Check sheet for the modelled part. Datum: model origin and axes. Units: mm. Face numbers are marked on the shaded views. A direction names the side the tool comes from. Round coordinates to 2 decimals unless told otherwise and drop trailing zeros. One line per item, written item: value.
from build123d import *

# Parameters (mm, degrees)
CUT_EXTRUDE1_DEPTH      = 5
CUT_EXTRUDE1_DEPTH_BACK = 20.845866419
SKETCH2_W               = 7
SKETCH2_H               = 11
SKETCH2_H_2             = 13
CUT_EXTRUDE2_DEPTH      = 20.845866419
CUT_EXTRUDE2_DEPTH_BACK = 20.845866419
SKETCH3_R               = 1
CUT_EXTRUDE4_START      = -7.009047527
CUT_EXTRUDE4_DEPTH      = 14.018095848
SKETCH6_R               = 0.5
CUT_EXTRUDE5_DEPTH      = 25.059476613
SKETCH7_W               = 6.999992022
SKETCH7_H               = 6
CUT_EXTRUDE6_DEPTH      = 23.402723679


with BuildPart() as part:
    # Sketch1 → Revolve1 (revolve)
    with BuildSketch(Plane(origin=(0, 0, 0), x_dir=(0, 0, -1), z_dir=(1, 0, 0))):
        with BuildLine():
            Line((0, 16), (0, -16))
            Line((0, -16), (7, -16))
            add(Edge.make_bspline(
                [(7, 16), (9.604722665, 1.227883705), (7, -16)],
                knots=[0, 0, 0, 1, 1, 1], degree=2))
            Line((7, 16), (0, 16))
        make_face()
    revolve(axis=Axis((0, 16, 0), (0, -1, 0)))

    # Sketch2 → Cut-Extrude1 (cut, two sides: drawn at the far end of the back side and taken through both)
    with BuildSketch(Plane(origin=(0, 0, 0), x_dir=(0, 0, -1), z_dir=(1, 0, 0)).offset(-CUT_EXTRUDE1_DEPTH_BACK)):
        with Locations((0, 10.5)):
            Rectangle(SKETCH2_W, SKETCH2_H)
        with Locations((0, -9.5)):
            Rectangle(SKETCH2_W, SKETCH2_H_2)
    extrude(amount=CUT_EXTRUDE1_DEPTH + CUT_EXTRUDE1_DEPTH_BACK, mode=Mode.SUBTRACT)

    # Sketch3 → Cut-Extrude2 (cut, two sides: drawn at the far end of the back side and taken through both)
    with BuildSketch(Plane.XY.offset(-CUT_EXTRUDE2_DEPTH_BACK)):
        with Locations((0.468911087, 11)):
            Circle(SKETCH3_R)
        with Locations((0.468911087, -14)):
            Circle(SKETCH3_R)
    extrude(amount=CUT_EXTRUDE2_DEPTH + CUT_EXTRUDE2_DEPTH_BACK, mode=Mode.SUBTRACT)

    # Cut-Extrude4: read off the stored shape, not the designer's step
    # Cut-Extrude4 outline → Cut-Extrude4 (cut)
    with BuildSketch(Plane.XY.offset(CUT_EXTRUDE4_START)):
        with BuildLine():
            ThreePointArc((7.691484865, -10.632025277), (5.737835213, -14.460501747), (1.724865718, -16))
            Line((1.724865718, -16), (9, -16))
            Line((9, -16), (9, -7))
            Line((9, -7), (8.076213925, -7))
            Line((8.076213925, -7), (7.691484865, -10.632025277))
        make_face()
        with BuildLine():
            Line((-6.062177826, -16), (0.910117982, -16))
            ThreePointArc((0.910117982, -16), (-4.452137657, -13.936852235), (-7.048611862, -8.811553614))
            ThreePointArc((-7.048611862, -8.811553614), (-7.04931897, -8.804588968), (-7.050019983, -8.797623705))
            Line((-7.050019983, -8.797623705), (-7.233336424, -7))
            Line((-7.233336424, -7), (-9, -7))
            Line((-9, -7), (-9, -15.999999999))
            Line((-9, -15.999999999), (-6.062177826, -16))
        make_face()
    extrude(amount=CUT_EXTRUDE4_DEPTH, mode=Mode.SUBTRACT)

    # Sketch6 → Cut-Extrude5 (cut, through all)
    with BuildSketch(Plane(origin=(0, 5, 0), x_dir=(1, 0, 0), z_dir=(0, 1, 0))):
        with Locations(Location((4, 0, 0), (0, 0, 270))):
            Circle(SKETCH6_R)
        with Locations(Location((-3, 0, 0), (0, 0, 270))):
            Circle(SKETCH6_R)
    extrude(amount=-CUT_EXTRUDE5_DEPTH, mode=Mode.SUBTRACT)

    # Sketch7 → Cut-Extrude6 (cut, through all)
    with BuildSketch(Plane.ZY.offset(-5)):
        with Locations((-3.989e-06, -13)):
            Rectangle(SKETCH7_W, SKETCH7_H)
    extrude(amount=-CUT_EXTRUDE6_DEPTH, mode=Mode.SUBTRACT)


solid = part.part
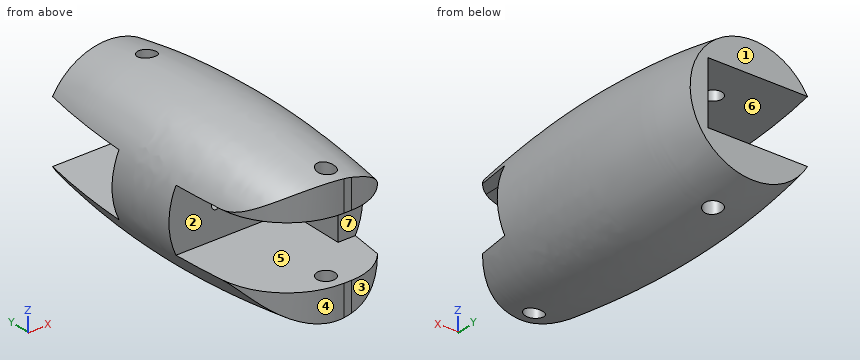
Q1. Sectioned sample at A-A on z = -6.25. State how many separate pieces and enclosed holes the cut face has, and give its area (3 significant figures).
Completed:
separate pieces: 1
enclosed holes: 2
area: 296 mm^2
Q2. Draft check along Z on the marked faces 1 and 2. Enter one of: pulls with the +Z half, pulls with the -Z half, needs draft (parallel to the pull), parting line crosses it, or undercut.
Completed:
face 1: needs draft
face 2: undercut
Q3. Access from +Z, -Z, +X, -X, +Y, -Y to the whole of each face (thin tool, end or side, straight path). Record for the marked faces 3, 4, 5, 6 and 7.
Completed:
face 3: +Z, -Z, +X, -Y
face 4: +Z, -Z, -X, -Y
face 5: -X, -Y
face 6: -X, +Y
face 7: +X, -X, -Y
Q4. Scan lines: line 1 (Y direction, x = -6, z = 1.75); line 2 (X direction, y = -14, z = -6.6); line 3 (X direction, y = 2.5, z = 0). Record each from-to range of solid material in increasing order. Write a range as [from, to].
Completed:
line 1: [-3, 5]
line 2: [-3.09, -0.53], [1.47, 3.09]
line 3: [-8.28, -3.5], [-2.5, 3.5], [4.5, 8.28]
Q5. Depth check by flat-ended pin: P1, Ø1.8, axis at x = 0.47, y = -14, coming from the -Z side; P2, Ø0.6, axis at x = 6, y = -12.5, coming from the -Z side; P3, Ø3.5, axis at x = 0, y = 13, coming from the +Z side; P4, Ø4, axis at y = -7, z = 2, coming from the -X side. Enter the tip coordinate at first touch or a pass-through.
Completed:
P1: through
P2: z = -4.85
P3: z = 7.67
P4: x = -7.31
